Geometry check sheet. Reference: the model listing, model coordinates, mm. A direction names the side the tool comes from. Give positions to 0.01 mm unless a question says otherwise; leave off trailing zeros. Write each loop counter-clockwise with the first axis right and the second up, starting at its lowest first coordinate (ties: lowest second). Pieces come first, ordered by that corner, then holes. Notation, with made-up numbers: (71, 46.25) - (96, 46.25) arc R9 ccw to (96, 59.25) - close; hole circle Ø8 at (-40, -17). An arc over 180 degrees is marked (long way). Write item = value, one per line. Start each with the question number.
(1) Section check B-B, the plane x = 23. Enter the section's corners in (y, z).
(2) Thickness scan on L1, parallel to Z at x = 64.5, y = 16; L2, parallel to X at y = -6, z = 25.5; L3, parallel to Z at x = 84, y = -5.5. Record the ranges inside material, lowest first.
(3) Access from +Z, -Z, +X, -X, +Y, -Y to the whole of each face (thin tool, end or side, straight path). Record for faces 1 (the flat face through (67, -27.5, 1)), 2 (the cylindrical face through (19.192, -21.029, 16.125)).
(4) Section check C-C, the plane z = 42. Enter the section's corners in (x, y).
(5) Section check A-A, the plane y = 0. Enter the section's corners in (x, z), plus the area to 3 significant figures.
(6) Depth check by flat-ended pin: pin 1 Ø4 at (x, y) = (26.5, 9) entering from -Z; pin 2 Ø3 at (x, y) = (76.5, -19.5) entering from -Z; pin 3 Ø2 at (y, z) = (-5.5, 7.5) entering from +X. Enter the tip coordinate at first touch or a pass-through.
Autodesk Inventor part; units mm, degrees
ref_plane "YZ Plane" through (0, 0, 0) normal (1, 0, 0) x (0, 1, 0)
ref_plane "XZ Plane" through (0, 0, 0) normal (0, 1, 0) x (-1, 0, 0)
ref_plane "XY Plane" through (0, 0, 0) normal (0, 0, 1) x (1, 0, 0)
sketch "Sketch1" plane through (0, 0, 0) normal (1, 0, 0) x (0, 1, 0)
  circle A0 centre (0, 0) radius 26.5
  dimension "d0" = 53
extrude "Extrusion1" add sketch "Sketch1" along normal blind 51
sketch "Sketch2" plane through (0, 0, 0) normal (0, 1, 0) x (-1, 0, 0)
  line L0 (-51, 26.5) -> (-51, -26.5)
  circle A0 centre (-51, 0) radius 48
  point P0 (0, 0)
  dimension "d3" = 96
extrude "Extrusion2" add sketch "Sketch2" along normal mid plane 55
move or copy body "Move Body1" bodies to move or copy 1 copy no translate (15, 0, 0)
properties part number "hip"
Model answer:
q1.outline = (-27.5, -21.33) - (-15.72, -21.33) arc R26.5 ccw to (15.72, -21.33) - (27.5, -21.33) - (27.5, 21.33) - (15.72, 21.33) arc R26.5 ccw to (-15.72, 21.33) - (-27.5, 21.33) - close
q2.L1 = -47.98 to 47.98
q2.L2 = 15 to 106.67
q2.L3 = -44.5 to 44.5
q3.face_1 = +Z, -Z, +X, -X, -Y
q3.face_2 = -X
q4.outline = (42.76, -27.5) - (89.24, -27.5) - (89.24, 27.5) - (42.76, 27.5) - close
q5.outline = (15, -26.5) - (25.98, -26.5) arc R48 ccw (long way) to (25.98, 26.5) - (15, 26.5) - close
q5.area = 7,530 mm²
q6.pin_1 = -29.96
q6.pin_2 = -47.15
q6.pin_3 = 113.56
